The listing builds one solid part. Answer for the finished solid, in the listing's coordinates (mm). Face numbers are marked on the shaded views. A direction names the side the tool comes from. Round coordinates to 2 decimals unless told otherwise and drop trailing zeros. Write each loop counter-clockwise with the first axis right and the second up, starting at its lowest first coordinate (ties: lowest second). Pieces come first, ordered by that corner, then holes.
(1) The mould has two halves that part along Y. Classify the marked faces 1, 2 and 3: +Y half, -Y half, draft (parallel to the pull), parting line (faces both ways), or undercut.
(2) Each of these flat-tipped pins is pushed along its axis until it touches: pin 1 Ø2 at (y, z) = (154, 4) entering from +X; pin 2 Ø5 at (x, z) = (82, 6.5) entering from -Y; pin 3 Ø3 at (x, y) = (141.5, 162) entering from -Z; pin 4 Ø5 at (x, z) = (156, 9) entering from +Y. Where does it stop, or does it pass through?
(3) A cutting plane is placed at A-A, the plane x = 124.5. Give the number of separate pieces and of enclosed holes in the cut face, and give its area (3 significant figures).
(4) For the marked faces 4 and 5, determine the directions among +Z, -Z, +X, -X, +Y, -Y from which every point of the face is accessible in a straight line to the end or side of a thin tool.
(5) A cutting plane is placed at C-C, the plane y = 180.5. Give the vertices of the cut face in (x, z), and give its area (3 significant figures).
(6) Find the intervals of material crossed by probe 1 along X at (y, z) = (146.5, 2.75); probe 2 along X at (y, z) = (138, 11.5); probe 3 along Y at (x, z) = (148.5, 7.5), in increasing order.
(7) A cutting plane is placed at B-B, the plane x = 70. Give the vertices of the cut face in (y, z).
from build123d import *

# Parameters (mm, degrees)
EXTRUDE_1_DEPTH = 13


with BuildPart() as part:
    # 草图1 → 凸台-拉伸1 (new body)
    with BuildSketch(Plane.XY):
        with BuildLine():
            Line((47.511484966, 142.033134461), (110.638937631, 102.207761638))
            ThreePointArc((110.638937631, 102.207761638), (114.665827011, 101.043744068), (118.692649861, 102.207991771))
            Line((118.692649861, 102.207991771), (152.521772353, 123.552557153))
            ThreePointArc((152.521772353, 123.552557153), (153.81505185, 124.925900716), (153.04891629, 126.649757061))
            Line((153.04891629, 126.649757061), (136.489129492, 137.165850219))
            ThreePointArc((136.489129492, 137.165850219), (135.492047357, 138.983315731), (136.494426509, 140.797865181))
            Line((136.494426509, 140.797865181), (148.334619381, 148.268463065))
            ThreePointArc((148.334619381, 148.268463065), (150.056794855, 148.643643111), (151.618362398, 147.826235477))
            Line((151.618362398, 147.826235477), (169.12186053, 136.710849803))
            ThreePointArc((169.12186053, 136.710849803), (171.033857417, 136.155053995), (172.945854303, 136.710849803))
            Line((172.945854303, 136.710849803), (181.18602163, 143.463793951))
            ThreePointArc((181.18602163, 143.463793951), (182.315098555, 145.518303295), (181.18602163, 147.572812638))
            Line((181.18602163, 147.572812638), (148.25303307, 168.486510374))
            ThreePointArc((148.25303307, 168.486510374), (145.550526458, 169.274236069), (142.84573367, 168.494396508))
            Line((142.84573367, 168.494396508), (103.370364428, 143.587318295))
            ThreePointArc((103.370364428, 143.587318295), (102.195954559, 141.45767708), (103.370375956, 139.328042221))
            Line((103.370375956, 139.328042221), (128.55687664, 124.67236247))
            add(Edge.make_bspline(
                [(104.659407223, 125.955435879), (107.630554524, 124.900634476), (112.429978189, 123.518860294), (120.55796174, 122.941026513), (125.679246688, 122.847455284), (128.55687664, 124.67236247)],
                knots=[0, 0, 0, 0, 0.387587107, 0.604017493, 1, 1, 1, 1], degree=3))
            Line((104.659407223, 125.955435879), (72.452510917, 144.69618768))
            ThreePointArc((72.452510917, 144.69618768), (72.002596111, 145.454480563), (72.410625454, 146.236109301))
            Line((72.410625454, 146.236109301), (82.149898801, 152.636203216))
            ThreePointArc((82.149898801, 152.636203216), (83.207924224, 152.95258239), (84.265790914, 152.635672874))
            Line((84.265790914, 152.635672874), (88.402902158, 149.914029293))
            ThreePointArc((88.402902158, 149.914029293), (90.083226665, 149.40103976), (91.774170174, 149.877861281))
            Line((91.774170174, 149.877861281), (132.907259914, 175.690631112))
            ThreePointArc((132.907259914, 175.690631112), (133.18297095, 176.334767089), (132.980807122, 177.005630354))
            Line((132.980807122, 177.005630354), (117.031500859, 188.303055623))
            ThreePointArc((117.031500859, 188.303055623), (113.835262941, 189.244329835), (110.639025024, 188.303055623))
            Line((110.639025024, 188.303055623), (47.48382646, 147.572951165))
            ThreePointArc((47.48382646, 147.572951165), (45.979061901, 144.795460967), (47.511484966, 142.033134461))
        make_face()
    extrude(amount=EXTRUDE_1_DEPTH)


solid = part.part
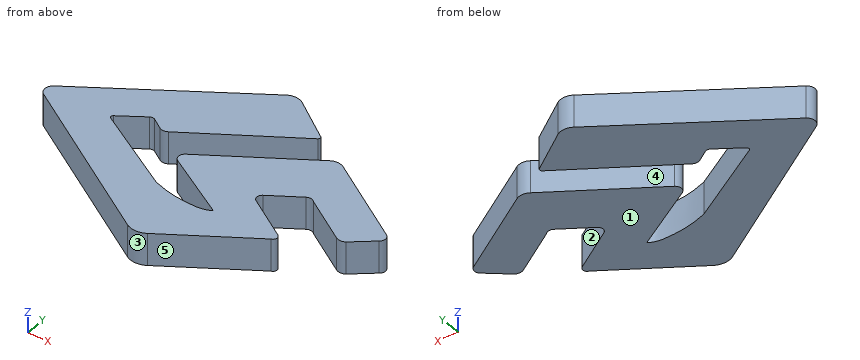
Solutions:
1. face 1: draft
1. face 2: undercut
1. face 3: -Y half
2. pin 1: stops at x = 172.64
2. pin 2: stops at y = 118.7
2. pin 3: stops at z = 0
2. pin 4: stops at y = 165.15
3. separate pieces: 3
3. enclosed holes: 0
3. area: 778 mm2
4. face 4: +Z, -Z
4. face 5: +Z, -Z, +X, -Y
5. outline: (98.54, 0) - (128.05, 0) - (128.05, 13) - (98.54, 13) - close
5. area: 384 mm2
6. probe 1: x = 46.45 to 72.81, 107.99 to 145.53, 153.71 to 182.11
6. probe 2: x = 53.9 to 83.96, 105.65 to 135.73, 167.09 to 174.52
6. probe 3: y = 121.02 to 129.54, 148.36 to 168.33
7. outline: (127.85, 0) - (162.09, 0) - (162.09, 13) - (127.85, 13) - close
